Check sheet for the drawn part. Datum: minimum x, y, z corner. Units: mm. Give positions to 0.01 mm unless a question says otherwise; leave off trailing zeros. Loops run counter-clockwise (first coordinate to the right, second up) from the corner with the lowest first, then second, coordinate; pieces in that order, holes last. Notation, with made-up numbers: (67, -38) - (80, -38) arc R27 ccw to (80, -19) - close; hole circle Ø10 at (44, 0.25). An arc over 180 degrees is marked (long way). Use one line per item in the form item = value.
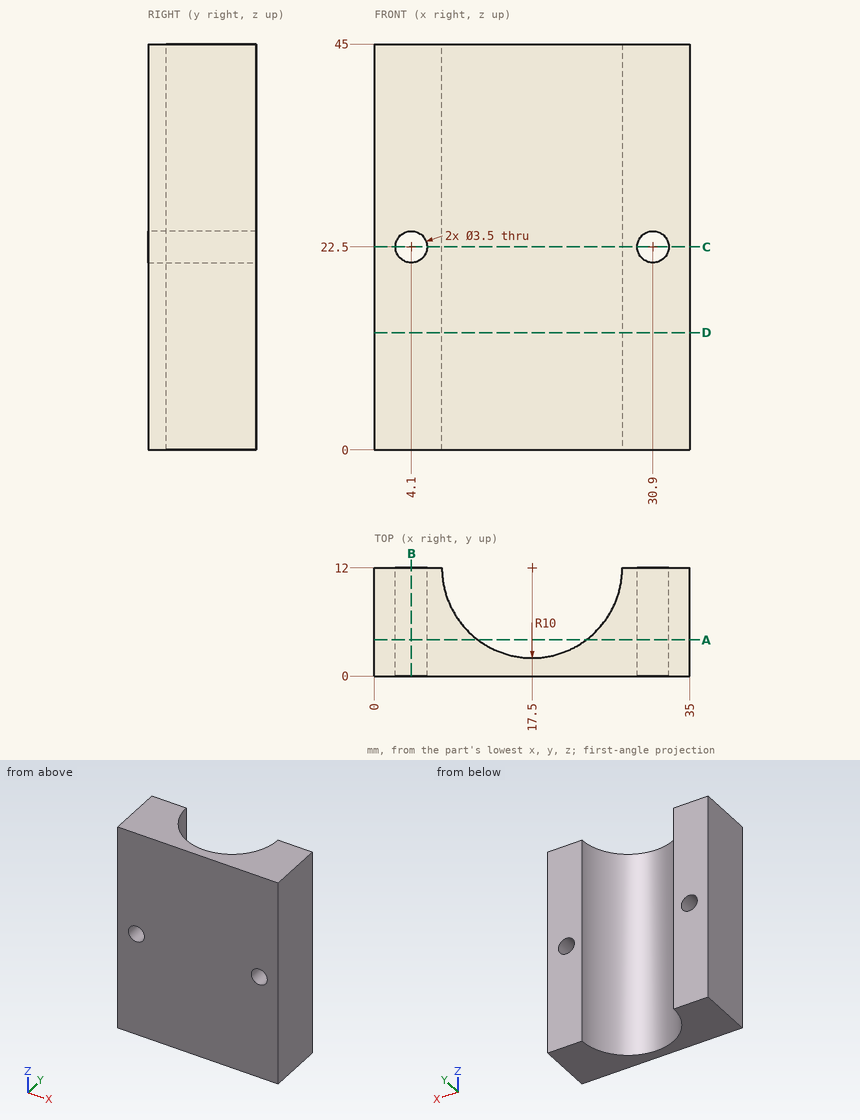
Item 1: Section check C-C on z = 22.5. Record the boundary of the cut face in (x, y), then the cut area to 3 significant figures.
Answer block:
outline = (0, 0) - (2.35, 0) - (2.35, 12) - (0, 12) - close; (5.85, 0) - (29.15, 0) - (29.15, 12) - (27.5, 12) arc R10 cw to (7.5, 12) - (5.85, 12) - close; (32.65, 0) - (35, 0) - (35, 12) - (32.65, 12) - close
area = 179 mm2
Item 2: Section check B-B on x = 4.1. Record the boundary of the cut face in (y, z).
Answer block:
outline = (0, 0) - (12, 0) - (12, 20.75) - (0, 20.75) - close; (0, 24.25) - (12, 24.25) - (12, 45) - (0, 45) - close
Item 3: Gauge pin test, flat end, axial feed: P1, Ø2, axis at x = 30.9, z = 22.5, coming from the +Y side. Record the tip position at first contact, or that the pin passes through.
Answer block:
P1 = through
Item 4: Thickness scan on L1, parallel to Z at x = 31, y = 6.25; L2, parallel to X at y = 7, z = 22; L3, parallel to X at y = 8.25, z = 22.5. Record the ranges inside material, lowest first.
Answer block:
L1 = 0 to 20.75, 24.25 to 45
L2 = 0 to 2.42, 5.78 to 8.84, 26.16 to 29.22, 32.58 to 35
L3 = 0 to 2.35, 5.85 to 8.23, 26.77 to 29.15, 32.65 to 35
Item 5: Section check D-D on z = 13. Record the boundary of the cut face in (x, y).
Answer block:
outline = (0, 0) - (35, 0) - (35, 12) - (27.5, 12) arc R10 cw to (7.5, 12) - (0, 12) - close
Item 6: Section check A-A on y = 4. Record the boundary of the cut face in (x, z), then the cut area to 3 significant figures.
Answer block:
outline = (0, 0) - (11.5, 0) - (11.5, 45) - (0, 45) - close; (23.5, 0) - (35, 0) - (35, 45) - (23.5, 45) - close; hole circle Ø3.5 at (4.1, 22.5); hole circle Ø3.5 at (30.9, 22.5)
area = 1,020 mm2
